Check sheet for the modelled part. Datum: model origin and axes. Units: mm. Face numbers are marked on the shaded views. A direction names the side the tool comes from. Round coordinates to 2 decimals unless told otherwise and drop trailing zeros. Write each loop counter-clockwise with the first axis right and the second up, starting at its lowest first coordinate (ties: lowest second). Pieces come first, ordered by that corner, then holes.
Item 1: Depth check by flat-ended pin: pin 1 (1.5 mm diameter, centred on y = 7, z = 30, fed in from +X); pin 2 (11 mm diameter, centred on x = 3.5, z = 29.5, fed in from +Y). Enter the tip coordinate at first touch or a pass-through.
Item 2: Material ranges on line 1 along Y through (x, z) = (402, 4); line 2 along Y through (x, z) = (244.5, 16), recorded low to high.
Item 3: Section check A-A, the plane z = 9. Record the cut outline in (x, y).
Item 4: Release check for a two-part mould opening along X. For the marked faces 3, 4 and 5 record: pulls with the +X half, pulls with the -X half, needs draft (parallel to the pull), parting line crosses it, or undercut.
Item 5: Section check C-C, the plane z = 35. Record the cut outline in (x, y), plus the area to 3 significant figures.
Item 6: Section check D-D, the plane x = 206. Record the cut outline in (y, z).
Item 7: Section check B-B, the plane y = 13.5. Record the cut outline in (x, z).
Item 8: Set-up check for the marked faces 1 and 2: record each of +Z, -Z, +X, -X, +Y, -Y from which the full face is reachable in a straight line by a thin tool's end or side.
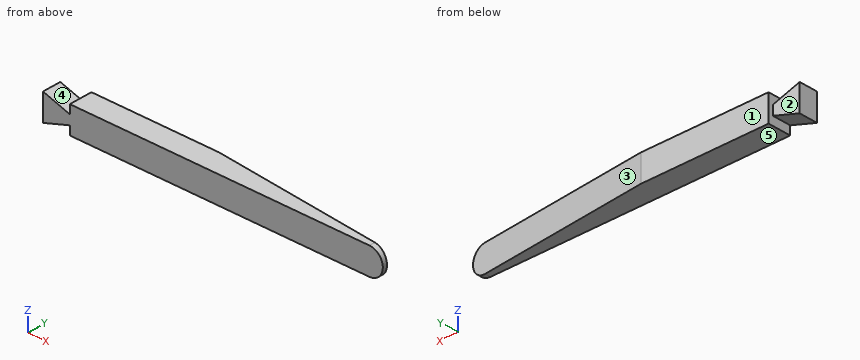
from build123d import *

# Parameters (mm, degrees)
BOSS_EXTRUDE1_DEPTH = 31.75
CUT_EXTRUDE2_DEPTH  = 442.504730683
CUT_EXTRUDE4_DEPTH  = 6.35


with BuildPart() as part:
    # Sketch2 → Boss-Extrude1 (new body)
    with BuildSketch(Plane(origin=(0, 0, 0), x_dir=(1, 0, 0), z_dir=(0, 1, 0))):
        with BuildLine():
            Line((14.300231201, -2.54), (420.689751691, -2.54))
            ThreePointArc((420.689751691, -2.54), (438.859641691, -20.70989), (420.689751691, -38.87978))
            Line((420.689751691, -38.87978), (14.300231201, -38.87978))
            Line((14.300231201, -38.87978), (14.300231201, -27.119548799))
            Line((14.300231201, -27.119548799), (-22.039548799, -38.87978))
            Line((-22.039548799, -38.87978), (-22.039548799, -2.54))
            Line((-22.039548799, -2.54), (14.300231201, -14.300231201))
            Line((14.300231201, -14.300231201), (14.300231201, -2.54))
        make_face()
    extrude(amount=BOSS_EXTRUDE1_DEPTH)

    # Sketch4 → Cut-Extrude2 (cut, through all)
    with BuildSketch(Plane.XY.offset(38.87978)):
        Polygon((187.5733876, 31.75), (438.859641691, 31.75), (438.859641691, 6.151225872), align=None)
    extrude(amount=-CUT_EXTRUDE2_DEPTH, mode=Mode.SUBTRACT)

    # Sketch8 → Cut-Extrude4 (cut)
    with BuildSketch(Plane(origin=(0, 31.75, 0), x_dir=(1, 0, 0), z_dir=(0, 1, 0))):
        Polygon((-22.039548799, -2.54), (14.300231201, -14.300231201), (14.300231201, -27.119548799), (-22.039548799, -38.87978), align=None)
    extrude(amount=-CUT_EXTRUDE4_DEPTH, mode=Mode.SUBTRACT)


solid = part.part
Values found:
1. pin 1: stops at x = 436.55
1. pin 2: stops at y = 25.4
2. line 1: y = 0 to 9.91
2. line 2: y = 0 to 25.95
3. outline: (-22.04, 0) - (-2.08, 0) - (-2.08, 25.4) - (-22.04, 25.4) - close; (14.3, 0) - (434.58, 0) - (434.58, 6.59) - (187.57, 31.75) - (14.3, 31.75) - close
4. face 3: pulls with the +X half
4. face 4: undercut
4. face 5: needs draft
5. outline: (-22.04, 0) - (-10.05, 0) - (-10.05, 25.4) - (-22.04, 25.4) - close; (14.3, 0) - (431.91, 0) - (431.91, 6.86) - (187.57, 31.75) - (14.3, 31.75) - close
5. area: 10,500 mm2
6. outline: (0, 2.54) - (29.87, 2.54) - (29.87, 38.88) - (0, 38.88) - close
7. outline: (-22.04, 2.54) - (14.3, 14.3) - (14.3, 2.54) - (366.72, 2.54) - (366.72, 38.88) - (14.3, 38.88) - (14.3, 27.12) - (-22.04, 38.88) - close
8. face 1: +Z, -Z, +X, -X, +Y
8. face 2: +Z, -Z, -X, +Y
